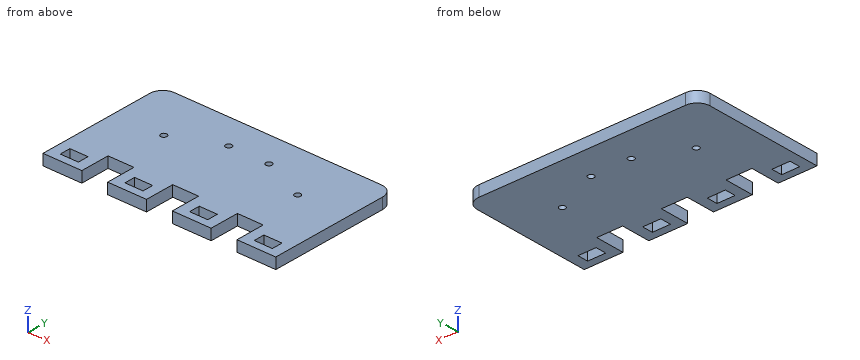
```python
from build123d import *

# Parameters (mm, degrees)
SKETCH1_W           = 114.3
SKETCH1_H           = 56.134
BOSS_EXTRUDE1_DEPTH = 5.334
SKETCH2_W           = 12.7
SKETCH2_H           = 5.334
CUT_EXTRUDE1_DEPTH  = 90.417531181
FILLET1_R           = 6.35
SKETCH3_R           = 1.5
CUT_EXTRUDE2_DEPTH  = 90.417531181
SKETCH4_W           = 19.05
SKETCH4_H           = 5.334
BOSS_EXTRUDE2_DEPTH = 9.144
SKETCH6_W           = 8.89
SKETCH6_H           = 5.334
CUT_EXTRUDE3_DEPTH  = 93.966642796


with BuildPart() as part:
    # Sketch1 → Boss-Extrude1 (new body)
    with BuildSketch(Plane.XY):
        with Locations((26.61749153, -2.755892293)):
            Rectangle(SKETCH1_W, SKETCH1_H)
    extrude(amount=BOSS_EXTRUDE1_DEPTH)

    # Sketch2 → Cut-Extrude1 (cut, through all)
    with BuildSketch(Plane.XY.offset(5.334)):
        with Locations((-5.13250847, -28.155892293)):
            Rectangle(SKETCH2_W, SKETCH2_H)
        with Locations((26.61749153, -28.155892293)):
            Rectangle(SKETCH2_W, SKETCH2_H)
        with Locations((58.36749153, -28.155892293)):
            Rectangle(SKETCH2_W, SKETCH2_H)
    extrude(amount=-CUT_EXTRUDE1_DEPTH, mode=Mode.SUBTRACT)

    # Fillet1
    fillet1_edges = [part.edges().sort_by_distance(p)[0] for p in [
        (-30.53250847, 25.311107707, 2.667),
        (83.76749153, 25.311107707, 2.667),
    ]]
    fillet(fillet1_edges, radius=FILLET1_R)

    # Sketch3 → Cut-Extrude2 (cut, through all)
    with BuildSketch(Plane(origin=(0, 0, 0), x_dir=(-1, 0, 0), z_dir=(0, 0, -1))):
        with Locations((6.24850847, -0.644892293)):
            Circle(SKETCH3_R)
        with Locations((-16.75149153, 9.355107707)):
            Circle(SKETCH3_R)
        with Locations((-59.48349153, -0.644892293)):
            Circle(SKETCH3_R)
        with Locations((-36.48349153, 9.355107707)):
            Circle(SKETCH3_R)
    extrude(amount=-CUT_EXTRUDE2_DEPTH, mode=Mode.SUBTRACT)

    # Sketch4 → Boss-Extrude2 (add)
    with BuildSketch(Plane(origin=(0, -30.822892293, 0), x_dir=(-1, 0, 0), z_dir=(0, -1, 0))):
        with Locations((-10.74249153, -2.667)):
            Rectangle(SKETCH4_W, SKETCH4_H)
        with Locations((21.00750847, -2.667)):
            Rectangle(SKETCH4_W, SKETCH4_H)
        with Locations((-42.49249153, -2.667)):
            Rectangle(SKETCH4_W, SKETCH4_H)
        with Locations((-74.24249153, -2.667)):
            Rectangle(SKETCH4_W, SKETCH4_H)
    extrude(amount=BOSS_EXTRUDE2_DEPTH)

    # Sketch6 → Cut-Extrude3 (cut, through all)
    with BuildSketch(Plane.XY.offset(5.334)):
        with Locations((-21.00750847, -33.489892293)):
            Rectangle(SKETCH6_W, SKETCH6_H)
        with Locations((10.74249153, -33.489892293)):
            Rectangle(SKETCH6_W, SKETCH6_H)
        with Locations((42.49249153, -33.489892293)):
            Rectangle(SKETCH6_W, SKETCH6_H)
        with Locations((74.24249153, -33.489892293)):
            Rectangle(SKETCH6_W, SKETCH6_H)
    extrude(amount=-CUT_EXTRUDE3_DEPTH, mode=Mode.SUBTRACT)


solid = part.part
```
Check sheet for the modelled part. Datum: model origin and axes. Units: mm. Round coordinates to 2 decimals unless told otherwise and drop trailing zeros. Write each loop counter-clockwise with the first axis right and the second up, starting at its lowest first coordinate (ties: lowest second). Pieces come first, ordered by that corner, then holes. Notation, with made-up numbers: (41.5, 29.25) -> (55.5, 29.25) arc R29 ccw to (55.5, 49.25) -> close; hole circle Ø4 at (-19.75, 49). An arc over 180 degrees is marked (long way). Put each result on its own line as item: value.
(1) Material ranges on line 1 (X direction, y = -29, z = 1.85); line 2 (X direction, y = 9.5, z = 0.35); line 3 (Y direction, x = 46, z = 1.2), recorded low to high.
Values found:
line 1: x = -30.53 to -11.48, 1.22 to 20.27, 32.97 to 52.02, 64.72 to 83.77
line 2: x = -30.53 to 15.26, 18.24 to 34.99, 37.98 to 83.77
line 3: y = -39.97 to -36.16, -30.82 to 25.31
(2) Go/stop test with a flat-tipped pin: pin 1 Ø2.5 at (x, z) = (29, 1.5) entering from -Y. Record where the tip stops, or that it passes through.
Values found:
pin 1: stops at y = -25.49
(3) Sectioned sample at B-B (z = 2.4). Count the separate pieces of the cut face and the enclosed holes in it, plus the area to 3 significant figures.
Values found:
separate pieces: 1
enclosed holes: 8
area: 6,670 mm^2
(4) Sectioned sample at A-A (x = 45). Enter the section's corners in (y, z), plus the area to 3 significant figures.
Values found:
outline: (-39.97, 0) -> (-36.16, 0) -> (-36.16, 5.33) -> (-39.97, 5.33) -> close; (-30.82, 0) -> (25.31, 0) -> (25.31, 5.33) -> (-30.82, 5.33) -> close
area: 320 mm^2
(5) Sectioned sample at C-C (x = -10). Enter the section's corners in (y, z), plus the area to 3 significant figures.
Values found:
outline: (-25.49, 0) -> (25.31, 0) -> (25.31, 5.33) -> (-25.49, 5.33) -> close
area: 271 mm^2
